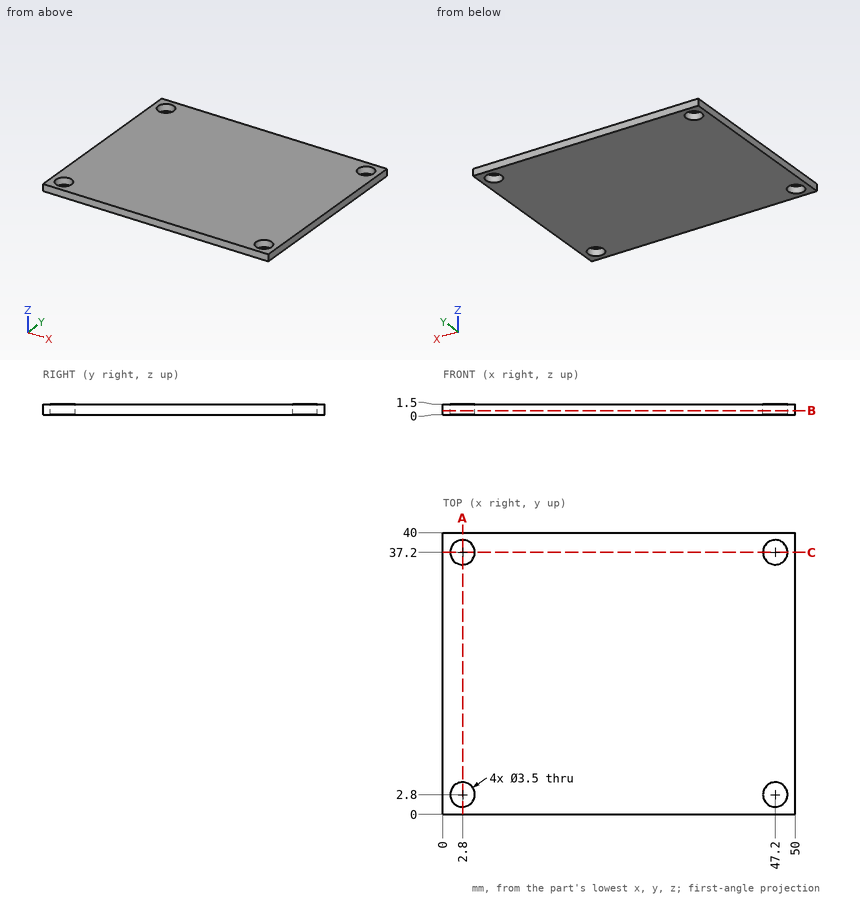
Print and shaded views of the part. All mm, measured from the part's lowest x, y and z. Coordinates: 2 decimals unless noted, no trailing zeros. Order: outer loops, then holes, each group sorted by start corner. A loop starts at its lowest first (then second) coordinate and runs counter-clockwise, first axis right, second up. Notation, with made-up numbers: (27.25, -20) - (67.25, -20) arc R17 cw to (67.25, -15) - close; hole circle Ø2 at (-35, -28). An arc over 180 degrees is marked (long way). Put each result on its own line as item: value.
1. Saw through at C-C (y = 37.2). Write the cut outline in (x, z), and give its area (3 significant figures).
Answer sheet:
outline: (0, 0) - (1.05, 0) - (1.05, 1.5) - (0, 1.5) - close; (4.55, 0) - (45.45, 0) - (45.45, 1.5) - (4.55, 1.5) - close; (48.95, 0) - (50, 0) - (50, 1.5) - (48.95, 1.5) - close
area: 64.5 mm^2
2. Probe line 1 along Y through (x, z) = (47.2, 1.2); line 2 along X through (y, z) = (37.2, 0.3). List the from-to ranges inside material, lowest first. Write a range as [from, to].
Answer sheet:
line 1: y = [0, 1.05], [4.55, 35.45], [38.95, 40]
line 2: x = [0, 1.05], [4.55, 45.45], [48.95, 50]
3. Saw through at B-B (z = 0.55). Write the cut outline in (x, y), and give its area (3 significant figures).
Answer sheet:
outline: (0, 0) - (50, 0) - (50, 40) - (0, 40) - close; hole circle Ø3.5 at (2.8, 2.8); hole circle Ø3.5 at (2.8, 37.2); hole circle Ø3.5 at (47.2, 2.8); hole circle Ø3.5 at (47.2, 37.2)
area: 1,960 mm^2
4. Saw through at A-A (x = 2.8). Write the cut outline in (y, z).
Answer sheet:
outline: (0, 0) - (1.05, 0) - (1.05, 1.5) - (0, 1.5) - close; (4.55, 0) - (35.45, 0) - (35.45, 1.5) - (4.55, 1.5) - close; (38.95, 0) - (40, 0) - (40, 1.5) - (38.95, 1.5) - close
